Check sheet for the modelled part. Datum: model origin and axes. Units: mm. Face numbers are marked on the shaded views. A direction names the side the tool comes from. Give positions to 0.01 mm unless a question says otherwise; leave off trailing zeros. Order: outer loops, then holes, each group sorted by start corner. A loop starts at its lowest first (then second) coordinate and runs counter-clockwise, first axis right, second up. Notation, with made-up numbers: (13.25, -15.5) -> (59.25, -15.5) arc R19 ccw to (59.25, 8.5) -> close; hole circle Ø10 at (64.25, -6). An arc over 180 degrees is marked (long way). Answer in a Markdown table with one row per item. Add a question column.
(1) Cross-section at B-B (x = 119.5). Record the cut outline in (y, z), then the cut area to 3 significant figures.
(2) Go/stop test with flat-tipped pins: pin 1 (12 mm diameter, centred on x = 20, z = 17, fed in from +Y); pin 2 (10 mm diameter, centred on x = -14.5, z = 9, fed in from +Y); pin 3 (1.5 mm diameter, centred on x = 76, y = 71, fed in from +Z); pin 4 (4 mm diameter, centred on x = 78.5, z = 2.5, fed in from -Y). Record where each tip stops, or that it passes through.
(3) Thickness scan on L1, parallel to X at y = 65.5, z = 8.5; L2, parallel to X at y = 70, z = 7.5; L3, parallel to X at y = 98, z = 9.25. Record the ranges inside material, lowest first. Write a range as [from, to].
(4) Release check for a two-part mould opening along X. For the marked faces 1, 2, 3 and 4 record: released by +X, released by -X, zero draft, split by the parting line, or undercut.
(5) Set-up check for the marked faces 5 and 6: record each of +Z, -Z, +X, -X, +Y, -Y from which the full face is reachable in a straight line by a thin tool's end or side.
(6) Cross-section at A-A (y = 7.5). Record the cut outline in (x, z).
```python
from build123d import *

# Parameters (mm, degrees)
BOSS_EXTRU_2_DEPTH      = 20
ESQUISSE4_W             = 5
ESQUISSE4_H             = 20
ENL_V_MAT_EXTRU_1_DEPTH = 10


with BuildPart() as part:
    # Esquisse2 → Boss.-Extru.2 (new body)
    with BuildSketch(Plane.XY):
        Polygon((0, 0), (-20, 0), (-20, 34.641016151), (0, 34.641016151), (129.903810568, 109.641016151), (149.903810568, 109.641016151), (149.903810568, 0), (129.37876344, 0), (129.37876344, 74.696863899), align=None)
    extrude(amount=BOSS_EXTRU_2_DEPTH)

    # Esquisse4 → Enlèv. mat.-Extru.1 (cut)
    with BuildSketch(Plane(origin=(-15, 25.980762114, 0), x_dir=(0.8660254037844379, 0.5000000000000013, 0), z_dir=(-0.5000000000000013, 0.8660254037844379, 0))):
        with Locations((24.820508076, -10)):
            Rectangle(ESQUISSE4_W, ESQUISSE4_H)
        with Locations((39.820508076, -10)):
            Rectangle(ESQUISSE4_W, ESQUISSE4_H)
        with Locations((54.820508076, -10)):
            Rectangle(ESQUISSE4_W, ESQUISSE4_H)
        with Locations((69.820508076, -10)):
            Rectangle(ESQUISSE4_W, ESQUISSE4_H)
        with Locations((84.820508076, -10)):
            Rectangle(ESQUISSE4_W, ESQUISSE4_H)
        with Locations((99.820508076, -10)):
            Rectangle(ESQUISSE4_W, ESQUISSE4_H)
        with Locations((114.820508076, -10)):
            Rectangle(ESQUISSE4_W, ESQUISSE4_H)
        with Locations((129.820508076, -10)):
            Rectangle(ESQUISSE4_W, ESQUISSE4_H)
        with Locations((144.820508076, -10)):
            Rectangle(ESQUISSE4_W, ESQUISSE4_H)
        with Locations((159.820508076, -10)):
            Rectangle(ESQUISSE4_W, ESQUISSE4_H)
    extrude(amount=-ENL_V_MAT_EXTRU_1_DEPTH, mode=Mode.SUBTRACT)


solid = part.part
```
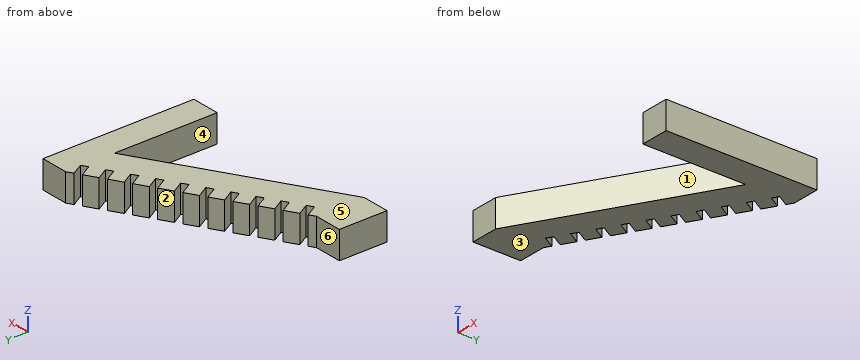
Answer below:
| question | item | result |
|---|---|---|
| 1 | outline | (68.99, 0) -> (103.63, 0) -> (103.63, 20) -> (68.99, 20) -> close |
| 1 | area | 693 mm² |
| 2 | pin 1 | stops at y = 49.65 |
| 2 | pin 2 | stops at y = 34.64 |
| 2 | pin 3 | passes through |
| 2 | pin 4 | stops at y = 44.17 |
| 3 | L1 | x = [53.45, 57.24], [63.01, 113.45], [129.38, 149.9] |
| 3 | L2 | x = [61.24, 71.96], [77.74, 121.24], [129.38, 149.9] |
| 3 | L3 | x = [113.53, 125.08], [129.74, 149.9] |
| 4 | face 1 | undercut |
| 4 | face 2 | released by -X |
| 4 | face 3 | zero draft |
| 4 | face 4 | undercut |
| 5 | face 5 | +Z, +X, -X, +Y, -Y |
| 5 | face 6 | +Z, -Z, -X, +Y |
| 6 | outline | (-20, 0) -> (12.99, 0) -> (12.99, 20) -> (-20, 20) -> close; (129.38, 0) -> (149.9, 0) -> (149.9, 20) -> (129.38, 20) -> close |
